```python
from build123d import *

# Parameters (mm, degrees)
SKETCH1_W           = 6.266
SKETCH1_H           = 19.6
SKETCH1_R           = 1.475
SKETCH1_W_2         = 52.832
SKETCH1_H_2         = 5
BOSS_EXTRUDE2_DEPTH = 3.175


with BuildPart() as part:
    # Sketch1 → Boss-Extrude2 (new body)
    # profile 1 of 4: a face of its own
    with BuildSketch(Plane.XY):
        with Locations((-23.283, 0)):
            Rectangle(SKETCH1_W, SKETCH1_H)
        with Locations((-23.95, -4.974)):
            Circle(SKETCH1_R, mode=Mode.SUBTRACT)
        with Locations((-23.95, 4.974)):
            Circle(SKETCH1_R, mode=Mode.SUBTRACT)
    # profile 2 of 4: a face of its own
    with BuildSketch(Plane.XY):
        with Locations((23.283, 0)):
            Rectangle(SKETCH1_W, SKETCH1_H)
        with Locations((23.95, -4.974)):
            Circle(SKETCH1_R, mode=Mode.SUBTRACT)
        with Locations((23.95, 4.974)):
            Circle(SKETCH1_R, mode=Mode.SUBTRACT)
    # profile 3 of 4: a face of its own
    with BuildSketch(Plane.XY):
        with Locations((0, 12.3)):
            Rectangle(SKETCH1_W_2, SKETCH1_H_2)
    # profile 4 of 4: a face of its own
    with BuildSketch(Plane.XY):
        with Locations((0, -12.3)):
            Rectangle(SKETCH1_W_2, SKETCH1_H_2)
    extrude(amount=BOSS_EXTRUDE2_DEPTH)


solid = part.part
```
Input: part model. Units: mm. Frame: model coordinates. A direction names the side the tool comes from. Round coordinates to 2 decimals unless told otherwise and drop trailing zeros. Order: outer loops, then holes, each group sorted by start corner. A loop starts at its lowest first (then second) coordinate and runs counter-clockwise, first axis right, second up. Notation, with made-up numbers: (8.25, 35.25) - (47.25, 35.25) arc R26 ccw to (47.25, 67.25) - close; hole circle Ø5 at (57.25, 5.5). An arc over 180 degrees is marked (long way). One line per question, with ' | ' between items. Start each with the question number.
1) Cut plane D-D, the plane x = 23.95. Return the cut outline in (y, z) (3 decimals), then the cut area to 3 significant figures.
2) Cut plane B-B, the plane y = 0. Return the cut outline in (x, z) (3 decimals), then the cut area to 3 significant figures.
3) Contact query for a flat-ended pin moving along its axis: P1, Ø2.5, axis at x = -23.95, y = -4.974, coming from the -Z side. Output: stop coordinate, or through.
4) Cut plane A-A, the plane x = 18. Return the cut outline in (y, z) (3 decimals).
5) Ray query, probe 1 along Y at (x, z) = (-23.95, 2.15); probe 2 along Y at (x, z) = (1, 1.5); probe 3 along X at (y, z) = (1.5, 1.95). Return the intervals inside material, ascending.
6) Set-up query: faces 4 (the flat face through (0, -9.8, 2)), 5 (the flat face through (0, 14.8, 2)). Return all of +Z, -Z, +X, -X, +Y, -Y with unobstructed straight access to the full face (end or side cutting, diameter ignored); none if empty.
7) Pull-direction query (X, two-part tool) for faces 1 (the flat face through (0, 9.8, 2)), 2 (the flat face through (-26.416, 0, 2)), 3 (the flat face through (0, 10, 3.175)); classes: +X half, -X half, draft (parallel to the pull), parting line (faces both ways), or undercut.
8) Cut plane C-C, the plane y = -4. Return the cut outline in (x, z) (3 decimals).
Worked out:
1) outline: (-14.8, 0) - (-6.449, 0) - (-6.449, 3.175) - (-14.8, 3.175) - close; (-3.499, 0) - (3.499, 0) - (3.499, 3.175) - (-3.499, 3.175) - close; (6.449, 0) - (14.8, 0) - (14.8, 3.175) - (6.449, 3.175) - close | area: 75.2 mm^2
2) outline: (-26.416, 0) - (-20.15, 0) - (-20.15, 3.175) - (-26.416, 3.175) - close; (20.15, 0) - (26.416, 0) - (26.416, 3.175) - (20.15, 3.175) - close | area: 39.8 mm^2
3) P1: passes through
4) outline: (-14.8, 0) - (-9.8, 0) - (-9.8, 3.175) - (-14.8, 3.175) - close; (9.8, 0) - (14.8, 0) - (14.8, 3.175) - (9.8, 3.175) - close
5) probe 1: y = -14.8 to -6.45, -3.5 to 3.5, 6.45 to 14.8 | probe 2: y = -14.8 to -9.8, 9.8 to 14.8 | probe 3: x = -26.42 to -20.15, 20.15 to 26.42
6) face 4: +Z, -Z | face 5: +Z, -Z, +X, -X, +Y
7) face 1: undercut | face 2: -X half | face 3: draft
8) outline: (-26.416, 0) - (-25.058, 0) - (-25.058, 3.175) - (-26.416, 3.175) - close; (-22.842, 0) - (-20.15, 0) - (-20.15, 3.175) - (-22.842, 3.175) - close; (20.15, 0) - (22.842, 0) - (22.842, 3.175) - (20.15, 3.175) - close; (25.058, 0) - (26.416, 0) - (26.416, 3.175) - (25.058, 3.175) - close
